```python
from build123d import *

# Parameters (mm, degrees)
F1_DEPTH = 27
F2_DEPTH = 18
F3_R     = 1.9999
F4_R     = 0.5


# Not quite as in the source:
# - a fillet or chamfer is up to 0.001 mm smaller than in the source, because OpenCascade refuses the exact size


with BuildPart() as f1:
    # F0 (on Top) → F1 (new body)
    with BuildSketch(Plane.XY):
        with BuildLine():
            ThreePointArc((6.6154708154, -2.2881315283), (4.8415745742, -5.0556063576), (2, -6.7082039325))
            ThreePointArc((2, -6.7082039325), (0, -7), (-2, -6.7082039325))
            ThreePointArc((-2, -6.7082039325), (-3.7888849897, 5.8859451692), (6.9342650073, -0.9570625938))
            Line((6.9342650073, -0.9570625938), (8.3233295817, 2.1638356393))
            ThreePointArc((8.3233295817, 2.1638356393), (5.7987889756, 6.3509091015), (1.4, 8.4852813742))
            Line((1.4, 8.4852813742), (1.4, 10.1))
            Line((1.4, 10.1), (-1.4, 10.1))
            Line((-1.4, 10.1), (-1.4, 8.4852813742))
            ThreePointArc((-1.4, 8.4852813742), (-4.8595970429, -7.0953728994), (8.4177416777, 1.7611431082))
            Line((8.4177416777, 1.7611431082), (6.6154708154, -2.2881315283))
        make_face()
    extrude(amount=F1_DEPTH)

    # F0 (on Top) → F2 (join)
    with BuildSketch(Plane.XY):
        with BuildLine():
            ThreePointArc((-2, -6.7082039325), (0, -7), (2, -6.7082039325))
            Line((2, -6.7082039325), (2, -5))
            Line((2, -5), (-2, -5))
            Line((-2, -5), (-2, -6.7082039325))
        make_face()
        with BuildLine():
            ThreePointArc((6.6154708154, -2.2881315283), (4.8415745742, -5.0556063576), (2, -6.7082039325))
            ThreePointArc((2, -6.7082039325), (0, -7), (-2, -6.7082039325))
            ThreePointArc((-2, -6.7082039325), (-3.7888849897, 5.8859451692), (6.9342650073, -0.9570625938))
            Line((6.9342650073, -0.9570625938), (8.3233295817, 2.1638356393))
            ThreePointArc((8.3233295817, 2.1638356393), (5.7987889756, 6.3509091015), (1.4, 8.4852813742))
            Line((1.4, 8.4852813742), (1.4, 10.1))
            Line((1.4, 10.1), (-1.4, 10.1))
            Line((-1.4, 10.1), (-1.4, 8.4852813742))
            ThreePointArc((-1.4, 8.4852813742), (-4.8595970429, -7.0953728994), (8.4177416777, 1.7611431082))
            Line((8.4177416777, 1.7611431082), (6.6154708154, -2.2881315283))
        make_face()
    extrude(amount=F2_DEPTH)

    # F3 (radius 2 in the source; OpenCascade refuses exactly that, so slightly less here)
    f3_edges = [f1.edges().sort_by_distance(p)[0] for p in [
        (2, -5.854102, 18),
        (-2, -5.854102, 18),
        (2, -5.854102, 0),
        (-2, -5.854102, 0),
    ]]
    fillet(f3_edges, radius=F3_R)

    # F4
    f4_edges = [f1.edges().sort_by_distance(p)[0] for p in [
        (2, -5, 9),
        (1.4, 10.1, 13.5),
        (-1.4, 10.1, 13.5),
    ]]
    fillet(f4_edges, radius=F4_R)


solid = f1.part
```
Work out the finished part from the listing and answer in its coordinate system (mm). A direction names the side the tool comes from. Give positions to 0.01 mm unless a question says otherwise; leave off trailing zeros. Write each loop counter-clockwise with the first axis right and the second up, starting at its lowest first coordinate (ties: lowest second). Pieces come first, ordered by that corner, then holes. Notation, with made-up numbers: (-27, -15) -> (14, -15) arc R11 ccw to (14, -7) -> close; hole circle Ø7 at (70.25, 30). An arc over 180 degrees is marked (long way). Write each question's results on one line, items separated by ' | '.
1. Find section B-B on z = 3. Determine the outline of the cut face in (x, y).
Data:
outline: (-2, -6.71) arc R7 cw (long way) to (6.93, -0.96) -> (8.32, 2.16) arc R8.6 ccw to (1.4, 8.49) -> (1.4, 9.6) arc R0.5 ccw to (0.9, 10.1) -> (-0.9, 10.1) arc R0.5 ccw to (-1.4, 9.6) -> (-1.4, 8.49) arc R8.6 ccw (long way) to (8.42, 1.76) -> (6.62, -2.29) arc R7 cw to (2, -6.71) -> (2, -5.5) arc R0.5 ccw to (1.5, -5) -> (-1.5, -5) arc R0.5 ccw to (-2, -5.5) -> close
2. Find section C-C on y = -3.75. Determine the outline of the cut face in (x, z).
Data:
outline: (-7.74, 0) -> (-5.91, 0) -> (-5.91, 27) -> (-7.74, 27) -> close; (5.91, 0) -> (7.74, 0) -> (7.74, 27) -> (5.91, 27) -> close
3. Determine the mould class of faces 1 (the flat face through (-4, 6, 27)), 2 (the flat face through (1.4, 9, 13)), 3 (the flat face through (2, -6, 9)) for opening direction X: +X half, -X half, draft (parallel to the pull), parting line (faces both ways), or undercut.
Data:
face 1: draft | face 2: +X half | face 3: undercut
4. Find section D-D on y = 0. Determine the outline of the cut face in (x, z).
Data:
outline: (-8.6, 0) -> (-7, 0) -> (-7, 27) -> (-8.6, 27) -> close; (7, 0) -> (7.36, 0) -> (7.36, 27) -> (7, 27) -> close; (7.63, 0) -> (8.6, 0) -> (8.6, 27) -> (7.63, 27) -> close
5. Straight lines are drawn through the part: L1, parallel to X at y = 1, z = 8.25; L2, parallel to X at y = 0, z = 12; L3, parallel to Y at x = 0, z = 8.75. For each, find the intervals that lie inside material, in ascending order.
Data:
L1: -8.54 to -6.93, 6.93 to 7.81, 8.08 to 8.54 | L2: -8.6 to -7, 7 to 7.36, 7.63 to 8.6 | L3: -8.6 to -5, 7 to 10.1
6. Each of these flat-tipped pins is pushed along its axis until it touches: pin 1 Ø6 at (x, y) = (1.5, -2.5) entering from -Z; pin 2 Ø5 at (x, z) = (5.5, 2.5) entering from +Y; pin 3 Ø1 at (y, z) = (-6, 11) entering from -X; pin 4 Ø1 at (x, y) = (-1, -3.5) entering from +Z. Where does it stop, or does it pass through?
Data:
pin 1: z = 0.09 | pin 2: y = 8.06 | pin 3: x = -6.61 | pin 4: through
7. Find section A-A on x = -3. Determine the outline of the cut face in (y, z), and give its area (3 significant figures).
Data:
outline: (-8.06, 0) -> (-6.32, 0) -> (-6.32, 27) -> (-8.06, 27) -> close; (6.32, 0) -> (8.06, 0) -> (8.06, 27) -> (6.32, 27) -> close | area: 93.7 mm^2
8. A tool of negligible diameter and unlimited length cuts with its end or side. For faces 4 (the flat face through (-1.4, 9, 13)), 5 (the cylindrical face through (5.85, 6.304, 13.311)), 6 (the cylindrical face through (1.43, -6.24, 0.6)), 7 (the cylindrical face through (-1.4, -6.26, 17.43)), 8 (the flat face through (0, -5, 9)), from which of +Z, -Z, +X, -X, +Y, -Y can it reach the whole face along a straight path? Write none if from no direction.
Data:
face 4: +Z, -Z, -X, +Y | face 5: +Z, -Z, +X, +Y | face 6: -Z | face 7: +Z | face 8: +Z, -Z
